from build123d import *

# Parameters (mm, degrees)
EXTRUDE_THIN3_DEPTH     = 3.1
SKETCH2_W               = 2.4
SKETCH2_H               = 1
CUT_EXTRUDE1_DEPTH      = 4.1
CUT_EXTRUDE1_DEPTH_BACK = 4.1
SKETCH3_W               = 2.4
SKETCH3_H               = 0.15
CUT_EXTRUDE2_DEPTH      = 1
FILLET1_R               = 0.15
SKETCH4_R               = 1.6
CUT_EXTRUDE3_DEPTH      = 1
EXTRUDE_THIN4_DEPTH     = 1
SKETCH6_W               = 1
SKETCH6_H               = 0.65
CUT_EXTRUDE4_DEPTH      = 0.5


with BuildPart() as part:
    # Sketch1 → Extrude-Thin3 (new body, symmetric)
    with BuildSketch(Plane(origin=(0, 0, 0), x_dir=(0, 0, -1), z_dir=(1, 0, 0))):
        Polygon((-3.1, 0.2), (-3.1, 2), (3.1, 2), (3.1, 0.2), (2.95, 0.2), (2.95, 1.85), (-2.95, 1.85), (-2.95, 0.2), align=None)
    extrude(amount=EXTRUDE_THIN3_DEPTH, both=True)

    # Sketch2 → Cut-Extrude1 (cut, two sides)
    with BuildSketch(Plane.XY) as cut_extrude1_sk:
        with Locations((0, 1.35)):
            Rectangle(SKETCH2_W, SKETCH2_H)
        Polygon((-3.1, 1.3), (-2, 0.2), (-3.1, 0.2), align=None)
        Polygon((3.1, 0.2), (3.1, 1.3), (2, 0.2), align=None)
    extrude(amount=CUT_EXTRUDE1_DEPTH, mode=Mode.SUBTRACT)
    extrude(cut_extrude1_sk.sketch, amount=-CUT_EXTRUDE1_DEPTH_BACK, mode=Mode.SUBTRACT)

    # Sketch3 → Cut-Extrude2 (cut)
    with BuildSketch(Plane(origin=(0, 2, 0), x_dir=(1, 0, 0), z_dir=(0, 1, 0))):
        with Locations((0, 3.025)):
            Rectangle(SKETCH3_W, SKETCH3_H)
        with Locations((0, -3.025)):
            Rectangle(SKETCH3_W, SKETCH3_H)
    extrude(amount=-CUT_EXTRUDE2_DEPTH, mode=Mode.SUBTRACT)

    # Fillet1
    fillet1_edges = [part.edges().sort_by_distance(p)[0] for p in [
        (-2.15, 2, -3.1),
        (2.15, 2, -3.1),
        (-2.15, 2, 3.1),
        (2.15, 2, 3.1),
    ]]
    fillet(fillet1_edges, radius=FILLET1_R)

    # Sketch4 → Cut-Extrude3 (cut)
    with BuildSketch(Plane(origin=(0, 2, 0), x_dir=(1, 0, 0), z_dir=(0, 1, 0))):
        Circle(SKETCH4_R)
    extrude(amount=-CUT_EXTRUDE3_DEPTH, mode=Mode.SUBTRACT)

    # Sketch5 → Extrude-Thin4 (add, symmetric)
    with BuildSketch(Plane.XY):
        with BuildLine():
            Line((3.1, 2), (3.4, 2))
            ThreePointArc((3.4, 2), (3.541421356, 1.941421356), (3.6, 1.8))
            Line((3.6, 1.8), (3.6, 0.35))
            ThreePointArc((3.6, 0.35), (3.658578644, 0.208578644), (3.8, 0.15))
            Line((3.8, 0.15), (4.2, 0.15))
            Line((4.2, 0.15), (4.2, 0))
            Line((4.2, 0), (3.8, 0))
            ThreePointArc((3.8, 0), (3.552512627, 0.102512627), (3.45, 0.35))
            Line((3.45, 0.35), (3.45, 1.8))
            ThreePointArc((3.45, 1.8), (3.435355339, 1.835355339), (3.4, 1.85))
            Line((3.4, 1.85), (3.1, 1.85))
            Line((3.1, 1.85), (3.1, 2))
        make_face()
    extrude(amount=EXTRUDE_THIN4_DEPTH, both=True)

    # Sketch6 → Cut-Extrude4 (cut)
    with BuildSketch(Plane.XZ):
        with Locations((3.7, 0.675)):
            Rectangle(SKETCH6_W, SKETCH6_H)
        with Locations((3.7, -0.675)):
            Rectangle(SKETCH6_W, SKETCH6_H)
    extrude(amount=-CUT_EXTRUDE4_DEPTH, mode=Mode.SUBTRACT)


solid = part.part
Verification items for the finished model (mm, model axes). Give positions to 0.01 mm unless a question says otherwise; leave off trailing zeros. Order: outer loops, then holes, each group sorted by start corner. A loop starts at its lowest first (then second) coordinate and runs counter-clockwise, first axis right, second up. Notation, with made-up numbers: (-23, 88.5) -> (-16, 88.5) arc R15 ccw to (-16, 107.5) -> close; hole circle Ø8 at (33, -18.5). An arc over 180 degrees is marked (long way). Answer as CSV lines item,"result".
Q1. Sectioned sample at C-C on z = 0. Record the cut outline in (x, y).
Solutions:
outline,"(-3.1, 1.85) -> (-1.6, 1.85) -> (-1.6, 2) -> (-3.1, 2) -> close; (1.6, 1.85) -> (3.4, 1.85) arc R0.05 cw to (3.45, 1.8) -> (3.45, 0.35) arc R0.35 ccw to (3.8, 0) -> (4.2, 0) -> (4.2, 0.15) -> (3.8, 0.15) arc R0.2 cw to (3.6, 0.35) -> (3.6, 1.8) arc R0.2 ccw to (3.4, 2) -> (1.6, 2) -> close"
Q2. Depth check by flat-ended pin: pin 1 (0.7 mm diameter, centred on y = 0.5, z = -0.5, fed in from -X). Enter the tip coordinate at first touch or a pass-through.
Solutions:
pin 1,"stops at x = 3.45"
Q3. Sectioned sample at B-B on y = 0.6. Record the cut outline in (x, z).
Solutions:
outline,"(-2.4, -3.1) -> (2.4, -3.1) -> (2.4, -2.95) -> (-2.4, -2.95) -> close; (-2.4, 2.95) -> (2.4, 2.95) -> (2.4, 3.1) -> (-2.4, 3.1) -> close; (3.45, -1) -> (3.6, -1) -> (3.6, 1) -> (3.45, 1) -> close"
Q4. Sectioned sample at A-A on y = 1.45. Record the cut outline in (x, z), plus the area to 3 significant figures.
Solutions:
outline,"(-3.1, -3.1) -> (-1.2, -3.1) -> (-1.2, -2.95) -> (-3.1, -2.95) -> close; (-3.1, 2.95) -> (-1.2, 2.95) -> (-1.2, 3.1) -> (-3.1, 3.1) -> close; (1.2, -3.1) -> (3.1, -3.1) -> (3.1, -2.95) -> (1.2, -2.95) -> close; (1.2, 2.95) -> (3.1, 2.95) -> (3.1, 3.1) -> (1.2, 3.1) -> close; (3.45, -1) -> (3.6, -1) -> (3.6, 1) -> (3.45, 1) -> close"
area,"1.44 mm²"
Q5. Scan lines: probe 1 along Z at (x, y) = (0, 1.95); probe 2 along X at (y, z) = (1.9, 0); probe 3 along Y at (x, z) = (-2.25, 3). Record each from-to range of solid material in increasing order.
Solutions:
probe 1,"z = -2.95 to -1.6, 1.6 to 2.95"
probe 2,"x = -3.1 to -1.6, 1.6 to 3.57"
probe 3,"y = 0.45 to 1.99"
Q6. Sectioned sample at D-D on x = 1. Record the cut outline in (y, z), plus the area to 3 significant figures.
Solutions:
outline,"(0.2, -3.1) -> (0.85, -3.1) -> (0.85, -2.95) -> (0.2, -2.95) -> close; (0.2, 2.95) -> (0.85, 2.95) -> (0.85, 3.1) -> (0.2, 3.1) -> close; (1.85, -2.95) -> (2, -2.95) -> (2, -1.25) -> (1.85, -1.25) -> close; (1.85, 1.25) -> (2, 1.25) -> (2, 2.95) -> (1.85, 2.95) -> close"
area,"0.705 mm²"
